Can you work these out from the drawing? Everything is in mm from the part's minimum corner. A direction names the side the tool comes from. Give positions to 0.01 mm unless a question says otherwise; leave off trailing zeros. Write each loop counter-clockwise with the first axis right and the second up, starting at its lowest first coordinate (ties: lowest second). Pieces come first, ordered by that corner, then holes. Notation, with made-up numbers: (37.25, 11) - (76.25, 11) arc R11 ccw to (76.25, 23) - close; hole circle Ø10 at (10.25, -38). An arc over 180 degrees is marked (long way). Use a Markdown table: item, result. Add a question column.
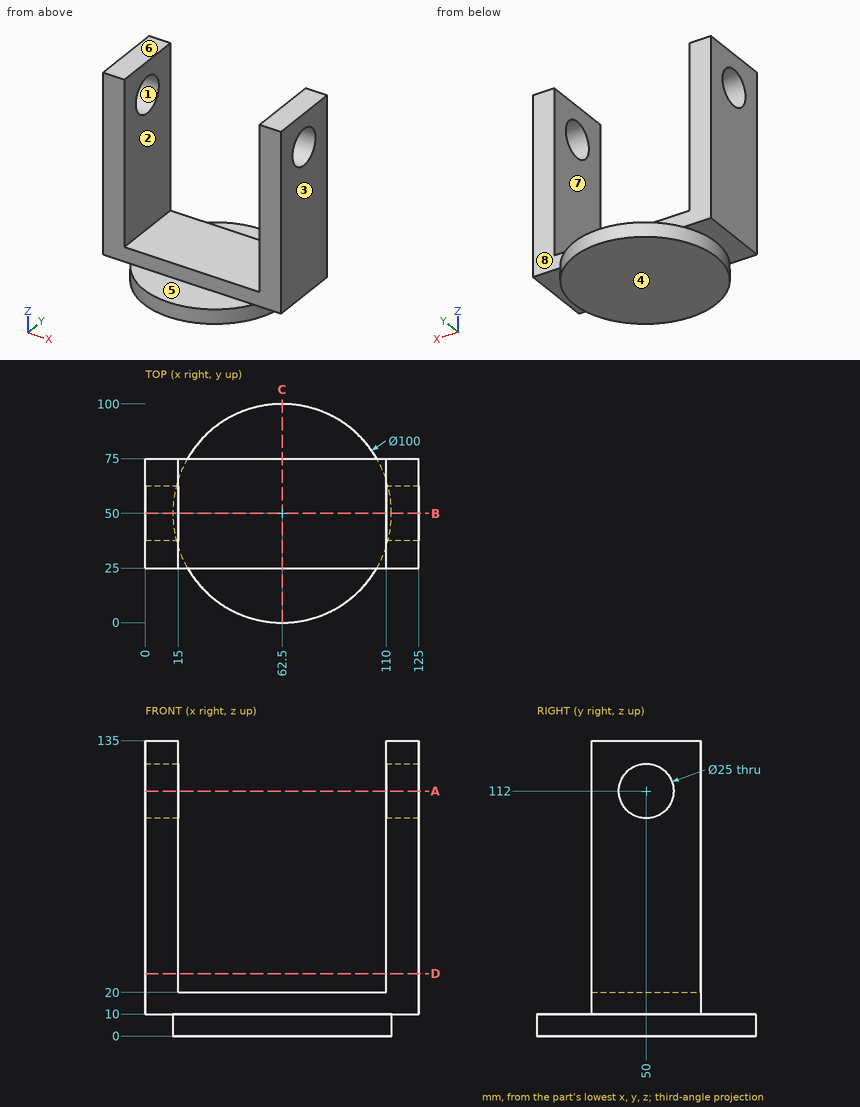
Q1. If we mould it in two halves opening along X, with no side actions, what happens to the marked faces 1, 2 and 3? For each: released by +X, released by -X, zero draft, split by the parting line, or undercut.
Q2. On a 3-axis mill with a long thin cutter (end or side, diameter ignored), from which of +Z, -Z, +X, -X, +Y, -Y can I reach the whole of each face in a straight line? I mean the marked faces 4, 5, 6, 7 and 8. Say none if no direction works.
Q3. Suppose I cut it at C-C (x = 62.5). Please give me the cut outline in (y, z), and give its area (3 significant figures).
Q4. Suppose I cut it at D-D (z = 28.5). Please give me the cut outline in (x, y).
Q5. Suppose I cut it at A-A (z = 112). Please give me the cut outline in (x, y).
Q6. I'm going to push flat-ended pins straight in: P1, Ø6, axis at x = 115.5, y = 40, coming from the -Z side; P2, Ø15, axis at x = 82, y = 37.5, coming from the +Z side; P3, Ø3, axis at x = 52.5, y = 80, coming from the +Z side. Where does each tip first touch, or does it pass through?
Q7. Suppose I cut it at B-B (y = 50). Please give me the cut outline in (x, z).
Q8. If I drill on probe 1 along Y at (x, z) = (10, 112); probe 2 along X at (y, z) = (65, 39); probe 3 along Z at (x, y) = (93, 87), over which ranges is the centre line in solid material (lowest first)? Write a range as [from, to].
Derived:
| question | item | result |
|---|---|---|
| 1 | face 1 | zero draft |
| 1 | face 2 | undercut |
| 1 | face 3 | released by +X |
| 2 | face 4 | -Z, +X, -X, +Y, -Y |
| 2 | face 5 | +Z, +X, -X, -Y |
| 2 | face 6 | +Z, +X, -X, +Y, -Y |
| 2 | face 7 | +Z, +Y, -Y |
| 2 | face 8 | +Z, +X, -X, +Y |
| 3 | outline | (0, 0) - (100, 0) - (100, 10) - (75, 10) - (75, 20) - (25, 20) - (25, 10) - (0, 10) - close |
| 3 | area | 1,500 mm² |
| 4 | outline | (0, 25) - (15, 25) - (15, 75) - (0, 75) - close; (110, 25) - (125, 25) - (125, 75) - (110, 75) - close |
| 5 | outline | (0, 25) - (15, 25) - (15, 37.5) - (0, 37.5) - close; (0, 62.5) - (15, 62.5) - (15, 75) - (0, 75) - close; (110, 25) - (125, 25) - (125, 37.5) - (110, 37.5) - close; (110, 62.5) - (125, 62.5) - (125, 75) - (110, 75) - close |
| 6 | P1 | z = 10 |
| 6 | P2 | z = 20 |
| 6 | P3 | z = 10 |
| 7 | outline | (0, 10) - (12.5, 10) - (12.5, 0) - (112.5, 0) - (112.5, 10) - (125, 10) - (125, 99.5) - (110, 99.5) - (110, 20) - (15, 20) - (15, 99.5) - (0, 99.5) - close; (0, 124.5) - (15, 124.5) - (15, 135) - (0, 135) - close; (110, 124.5) - (125, 124.5) - (125, 135) - (110, 135) - close |
| 8 | probe 1 | [25, 37.5], [62.5, 75] |
| 8 | probe 2 | [0, 15], [110, 125] |
| 8 | probe 3 | [0, 10] |
